Geometry check sheet. Reference: the model listing, model coordinates, mm. A direction names the side the tool comes from. Give positions to 0.01 mm unless a question says otherwise; leave off trailing zeros. Write item = value, one per line. Start each with the question number.
1. Cross-section at A-A, the plane x = 0. State how many separate pieces and enclosed holes the cut face has, plus the area to 3 significant figures.
2. Thickness scan on line 1 along Y through (x, z) = (9, 7); line 2 along X through (y, z) = (-20, 8.75); line 3 along X through (y, z) = (-15.5, 6). Record the ranges inside material, lowest first.
3. Depth check by flat-ended pin: P1, Ø2, axis at x = 13.5, z = 1.5, coming from the +Y side; P2, Ø3, axis at y = -4, z = 4, coming from the +X side; P3, Ø8, axis at x = -1, y = 8.5, coming from the +Z side; P4, Ø4, axis at x = -13.5, z = 6.5, coming from the +Y side. Enter the tip coordinate at first touch or a pass-through.
4. Set-up check for faces 4 (the cylindrical face through (-14.49, 20.28, 8.8)), 5 (the flat face through (20.2, 2.2, 4.7)): record each of +Z, -Z, +X, -X, +Y, -Y from which the full face is reachable in a straight line by a thin tool's end or side.
5. Mould release check, pull along Y, two halves, no side actions. Record for faces 1 (the cylindrical face through (-14.49, 20.279, 0.724)), 2 (the flat face through (-15.036, -13.645, 4.696)), 3 (the cylindrical face through (23.642, -7.889, 0.724)): pulls with the +Y half, pulls with the -Y half, needs draft (parallel to the pull), parting line crosses it, or undercut.
```python
from build123d import *

# Parameters (mm, degrees)
F0_R        = 14.2875
F1_DEPTH    = 9.525
F2_SIZE     = 8.0772
F3_T1_DEPTH = 33.8699635206
F3_T3_DEPTH = 33.8699635206
F3_T5_DEPTH = 33.8699635206
F3_T7_DEPTH = 33.8699635206
F3_T9_DEPTH = 33.8699635206
F4_T1_DEPTH = 33.8699635206
F4_T3_DEPTH = 33.8699635206
F4_T5_DEPTH = 33.8699635206
F4_T7_DEPTH = 33.8699635206
F4_T9_DEPTH = 33.8699635206


# Not quite as in the source:
# - a fillet or chamfer that OpenCascade refuses, or shapes differently, is made with other operations: its cross-section is extruded or revolved along the edge and cut away or added


with BuildPart() as f1:
    # F0 (on Top) → F1 (new body)
    with BuildSketch(Plane.XY):
        Polygon((30.1960443924, 9.8112895714), (0, 31.75), (-30.1960443924, 9.8112895714), (-18.6621817603, -25.6862895714), (18.6621817603, -25.6862895714), align=None)
        Polygon((-18.087352426, -20.2171537862), (-17.5125230918, -14.7480180011), (-12.4886978979, -12.5112669148), (-8.0397020384, -15.7436516137), (-8.6145313726, -21.2127873989), (-13.6383565665, -23.4495384851), align=None, mode=Mode.SUBTRACT)
        Circle(F0_R, mode=Mode.SUBTRACT)
        Polygon((13.6383565665, -23.4495384851), (8.6145313726, -21.2127873989), (8.0397020384, -15.7436516137), (12.4886978979, -12.5112669148), (17.5125230918, -14.7480180011), (18.087352426, -20.2171537862), align=None, mode=Mode.SUBTRACT)
        Polygon((-24.8169551322, 10.9546502895), (-19.4378658721, 12.0980110075), (-15.7581418145, 8.011263418), (-17.4575070171, 2.7811551105), (-22.8365962772, 1.6377943925), (-26.5163203348, 5.7245419819), align=None, mode=Mode.SUBTRACT)
        Polygon((-5.499261314, 22.225), (-2.749630657, 26.9875), (2.749630657, 26.9875), (5.499261314, 22.225), (2.749630657, 17.4625), (-2.749630657, 17.4625), align=None, mode=Mode.SUBTRACT)
        Polygon((26.5163203348, 5.7245419819), (22.8365962772, 1.6377943925), (17.4575070171, 2.7811551105), (15.7581418145, 8.011263418), (19.4378658721, 12.0980110075), (24.8169551322, 10.9546502895), align=None, mode=Mode.SUBTRACT)
    extrude(amount=F1_DEPTH)

    # F2
    f2_edges = [f1.edges().sort_by_distance(p)[0] for p in [
        (-18.662182, -25.68629, 4.7625),
        (18.662182, -25.68629, 4.7625),
        (30.196044, 9.81129, 4.7625),
        (0, 31.75, 4.7625),
        (-30.196044, 9.81129, 4.7625),
    ]]
    chamfer(f2_edges, length=F2_SIZE)

    # F3: fillet of radius 2.54 on 5 edges, made by hand

    # F3_s2 → F3_t1 (cut)
    with BuildSketch(Plane(origin=(-5.2331971634, -16.1061247565, 0), x_dir=(0, 0, 1), z_dir=(0.3090169944, 0.9510565163, 0))):
        with BuildLine():
            ThreePointArc((9.525, 23.1462895714), (8.7810512242, 24.9423407956), (6.985, 25.6862895714))
            Line((6.985, 25.6862895714), (9.525, 25.6862895714))
            Line((9.525, 25.6862895714), (9.525, 23.1462895714))
        make_face()
    extrude(amount=F3_T1_DEPTH, mode=Mode.SUBTRACT)

    # F3_s4 → F3_t3 (cut)
    with BuildSketch(Plane.YZ.offset(-16.9349817603)):
        with BuildLine():
            ThreePointArc((-23.1462895714, 9.525), (-24.9423407956, 8.7810512242), (-25.6862895714, 6.985))
            Line((-25.6862895714, 6.985), (-25.6862895714, 9.525))
            Line((-25.6862895714, 9.525), (-23.1462895714, 9.525))
        make_face()
    extrude(amount=F3_T3_DEPTH, mode=Mode.SUBTRACT)

    # F3_s6 → F3_t5 (cut)
    with BuildSketch(Plane(origin=(-5.2331971634, 16.1061247565, 0), x_dir=(0, 0, 1), z_dir=(0.3090169944, -0.9510565163, 0))):
        with BuildLine():
            ThreePointArc((9.525, 23.1462895714), (8.7810512242, 24.9423407956), (6.985, 25.6862895714))
            Line((6.985, 25.6862895714), (9.525, 25.6862895714))
            Line((9.525, 25.6862895714), (9.525, 23.1462895714))
        make_face()
    extrude(amount=F3_T5_DEPTH, mode=Mode.SUBTRACT)

    # F3_s8 → F3_t7 (cut)
    with BuildSketch(Plane(origin=(13.7006880435, 9.9541325265, 0), x_dir=(0, 0, 1), z_dir=(-0.8090169944, -0.5877852523, 0))):
        with BuildLine():
            ThreePointArc((9.525, 23.1462895714), (8.7810512242, 24.9423407956), (6.985, 25.6862895714))
            Line((6.985, 25.6862895714), (9.525, 25.6862895714))
            Line((9.525, 25.6862895714), (9.525, 23.1462895714))
        make_face()
    extrude(amount=F3_T7_DEPTH, mode=Mode.SUBTRACT)

    # F3_s10 → F3_t9 (cut)
    with BuildSketch(Plane(origin=(13.7006880435, -9.9541325265, 0), x_dir=(0, 0, 1), z_dir=(-0.8090169944, 0.5877852523, 0))):
        with BuildLine():
            ThreePointArc((6.985, 25.6862895714), (8.7810512242, 24.9423407956), (9.525, 23.1462895714))
            Line((9.525, 23.1462895714), (9.525, 25.6862895714))
            Line((9.525, 25.6862895714), (6.985, 25.6862895714))
        make_face()
    extrude(amount=F3_T9_DEPTH, mode=Mode.SUBTRACT)

    # F4: fillet of radius 2.54 on 5 edges, made by hand

    # F4_s2 → F4_t1 (cut)
    with BuildSketch(Plane(origin=(-5.2331971634, -16.1061247565, 0), x_dir=(0, 0, 1), z_dir=(0.3090169944, 0.9510565163, 0))):
        with BuildLine():
            ThreePointArc((0, 23.1462895714), (0.7439487758, 24.9423407956), (2.54, 25.6862895714))
            Line((2.54, 25.6862895714), (0, 25.6862895714))
            Line((0, 25.6862895714), (0, 23.1462895714))
        make_face()
    extrude(amount=F4_T1_DEPTH, mode=Mode.SUBTRACT)

    # F4_s4 → F4_t3 (cut)
    with BuildSketch(Plane.YZ.offset(-16.9349817603)):
        with BuildLine():
            ThreePointArc((-23.1462895714, 0), (-24.9423407956, 0.7439487758), (-25.6862895714, 2.54))
            Line((-25.6862895714, 2.54), (-25.6862895714, 0))
            Line((-25.6862895714, 0), (-23.1462895714, 0))
        make_face()
    extrude(amount=F4_T3_DEPTH, mode=Mode.SUBTRACT)

    # F4_s6 → F4_t5 (cut)
    with BuildSketch(Plane(origin=(13.7006880435, 9.9541325265, 0), x_dir=(0, 0, 1), z_dir=(-0.8090169944, -0.5877852523, 0))):
        with BuildLine():
            ThreePointArc((0, 23.1462895714), (0.7439487758, 24.9423407956), (2.54, 25.6862895714))
            Line((2.54, 25.6862895714), (0, 25.6862895714))
            Line((0, 25.6862895714), (0, 23.1462895714))
        make_face()
    extrude(amount=F4_T5_DEPTH, mode=Mode.SUBTRACT)

    # F4_s8 → F4_t7 (cut)
    with BuildSketch(Plane(origin=(13.7006880435, -9.9541325265, 0), x_dir=(0, 0, 1), z_dir=(-0.8090169944, 0.5877852523, 0))):
        with BuildLine():
            ThreePointArc((2.54, 25.6862895714), (0.7439487758, 24.9423407956), (0, 23.1462895714))
            Line((0, 23.1462895714), (0, 25.6862895714))
            Line((0, 25.6862895714), (2.54, 25.6862895714))
        make_face()
    extrude(amount=F4_T7_DEPTH, mode=Mode.SUBTRACT)

    # F4_s10 → F4_t9 (cut)
    with BuildSketch(Plane(origin=(-5.2331971634, 16.1061247565, 0), x_dir=(0, 0, 1), z_dir=(0.3090169944, -0.9510565163, 0))):
        with BuildLine():
            ThreePointArc((0, 23.1462895714), (0.7439487758, 24.9423407956), (2.54, 25.6862895714))
            Line((2.54, 25.6862895714), (0, 25.6862895714))
            Line((0, 25.6862895714), (0, 23.1462895714))
        make_face()
    extrude(amount=F4_T9_DEPTH, mode=Mode.SUBTRACT)


solid = f1.part
```
Answers:
q1.separate_pieces = 3
q1.enclosed_holes = 0
q1.area = 136 mm^2
q2.line_1 = -25.69 to -21.38, -15.05 to -11.1, 11.1 to 25.21
q2.line_2 = -18.41 to -18.06, -8.49 to 8.49, 18.06 to 18.41
q2.line_3 = -21.97 to -17.59, -8.38 to 8.38, 17.59 to 21.97
q3.P1 = 22.51
q3.P2 = 26.2
q3.P3 = through
q3.P4 = 23.39
q4.face_4 = +Z, -X, +Y
q4.face_5 = +Z, -Z
q5.face_1 = pulls with the +Y half
q5.face_2 = undercut
q5.face_3 = pulls with the -Y half
